from build123d import *

# Parameters (mm, degrees)
SKETCH1_R           = 1.4224
BOSS_EXTRUDE1_DEPTH = 31.75
SKETCH2_R           = 2.7051
BOSS_EXTRUDE2_DEPTH = 1.4986
FILLET1_R           = 1.016
CUT_EXTRUDE1_DEPTH  = 2.38125


with BuildPart() as part:
    # Sketch1 → Boss-Extrude1 (new body)
    with BuildSketch(Plane(origin=(0, 0, 0), x_dir=(1, 0, 0), z_dir=(0, 1, 0))):
        Circle(SKETCH1_R)
    extrude(amount=BOSS_EXTRUDE1_DEPTH)

    # Sketch2 → Boss-Extrude2 (add)
    with BuildSketch(Plane(origin=(0, 31.75, 0), x_dir=(1, 0, 0), z_dir=(0, 1, 0))):
        Circle(SKETCH2_R)
    extrude(amount=BOSS_EXTRUDE2_DEPTH)

    # Fillet1
    fillet1_edges = [part.edges().sort_by_distance(p)[0] for p in [
        (-2.7051, 33.2486, 0),
    ]]
    fillet(fillet1_edges, radius=FILLET1_R)

    # Sketch3 → Cut-Extrude1 (cut)
    with BuildSketch(Plane(origin=(0, 33.2486, 0), x_dir=(1, 0, 0), z_dir=(0, 1, 0))):
        Polygon((0, 0.916543552), (-0.79375, 0.458271776), (-0.79375, -0.458271776), (0, -0.916543552), (0.79375, -0.458271776), (0.79375, 0.458271776), align=None)
    extrude(amount=-CUT_EXTRUDE1_DEPTH, mode=Mode.SUBTRACT)


solid = part.part
The model under review builds one solid part; all positions refer to its coordinate system, in mm. A direction names the side the tool comes from. Round coordinates to 2 decimals unless told otherwise and drop trailing zeros. Write each loop counter-clockwise with the first axis right and the second up, starting at its lowest first coordinate (ties: lowest second). Pieces come first, ordered by that corner, then holes. Notation, with made-up numbers: M -31,82 L 18,82 A25 ccw 18,106 Z; hole C 15,45 d8. An arc over 180 degrees is marked long. Answer as CSV lines item,"result". Start each with the question number.
Q1. Consider section A-A, the plane z = 0. Give the boundary of the cut face in (x, y), then the cut area to 3 significant figures.
Q2. Tool access review of faces 1 (the face through (-0.31, 15.65, 1.39)), 2 (the face through (0.794, 32, 0)), 3 (the face through (0, 0, 0)): name each direction out of +Z, -Z, +X, -X, +Y, -Y from which nothing blocks a thin tool from reaching the whole face with its end or side.
Q3. Wall thickness on line 1 along Y through (x, z) = (1.6, 0.15); line 2 along Y through (x, z) = (-0.75, 0.35); line 3 along Z through (x, y) = (-1, 31.5): over which ranges is each line inside the solid? List them lowest first.
Q4. Clearance check with flat-ended pins moving along their axes: P1, Ø1, axis at x = 0.5, z = 2, coming from the -Y side; P2, Ø1.5, axis at y = 19, z = -1, coming from the +X side. State where each tip first meets the part, or that it passes through.
Q5. Consider section B-B, the plane y = 15.5. Give the boundary of the cut face in (x, z).
Q6. The part is to be moulded in two halves that separate along X. For faces 4 (the face through (0, 30.867, 0)), 5 (the face through (2.58, 31.99, -0.81)), 6 (the face through (1.2, 31.75, 1.2)), say which applies: +X half, -X half, draft (parallel to the pull), parting line (faces both ways), or undercut.
Result set:
1,outline,"M -2.71,31.75 L -1.42,31.75 L -1.42,0 L 1.42,0 L 1.42,31.75 L 2.71,31.75 L 2.71,32.23 A1.02 ccw 1.69,33.25 L 0.79,33.25 L 0.79,30.87 L -0.79,30.87 L -0.79,33.25 L -1.69,33.25 A1.02 ccw -2.71,32.23 Z"
1,area,"94.2 mm²"
2,face 1,"-Y"
2,face 2,"+Y"
2,face 3,"+Z, -Z, +X, -X, -Y"
3,line 1,"y = 31.75 to 33.25"
3,line 2,"y = 0 to 30.87"
3,line 3,"z = -1.01 to 1.01"
4,P1,"stops at y = 31.75"
4,P2,"stops at x = 1.4"
5,outline,"C 0,0 d2.84"
6,face 4,"undercut"
6,face 5,"parting line"
6,face 6,"draft"
